Autodesk Inventor part; units mm, degrees
ref_plane "YZ Plane" through (0, 0, 0) normal (1, 0, 0) x (0, 1, 0)
ref_plane "XZ Plane" through (0, 0, 0) normal (0, 1, 0) x (-1, 0, 0)
ref_plane "XY Plane" through (0, 0, 0) normal (0, 0, 1) x (1, 0, 0)
sketch "Sketch1" plane through (0, 0, 0) normal (0, 0, 1) x (1, 0, 0)
  circle A0 centre (0, 0) radius 5.7
  dimension "d0" = 11.4
extrude "Extrusion1" add sketch "Sketch1" along normal blind 3
chamfer "Chamfer1" distance 0.8 angle 45 1 edges at (-5.7, 0, 3)
sketch "Sketch2" plane through (0, 0, 0) normal (0, 0, 1) x (1, 0, 0)
  circle A0 centre (0, 0) radius 2.9
  dimension "d6" = 5.8
extrude "Extrusion2" cut sketch "Sketch2" along normal blind 10
properties part number "Insert3mm"
CAD build for the part. Positions are in the model's coordinates, mm. Coordinates: 2 decimals unless noted, no trailing zeros. Loops run counter-clockwise (first coordinate to the right, second up) from the corner with the lowest first, then second, coordinate; pieces in that order, holes last. Notation, with made-up numbers: (86, 57) - (131, 57) arc R13 ccw to (131, 66) - close; hole circle Ø6 at (-15, 86.5). An arc over 180 degrees is marked (long way). Return JSON: item names as keys, results as strings.
1. Probe L1, parallel to Y at x = 0, z = 1.6; L2, parallel to Y at x = -1, z = 1.6; L3, parallel to X at y = 2.5, z = 0.4. List the from-to ranges inside material, lowest first. Write a range as from..to.
Result:
{"L1": "y = -5.7..-2.9, 2.9..5.7", "L2": "y = -5.61..-2.72, 2.72..5.61", "L3": "x = -5.12..-1.47, 1.47..5.12"}
2. Band-saw the part on A-A (y = 0). Give the cut face in (x, z).
Result:
{"outline": "(-5.7, 0) - (-2.9, 0) - (-2.9, 3) - (-4.9, 3) - (-5.7, 2.2) - close; (2.9, 0) - (5.7, 0) - (5.7, 2.2) - (4.9, 3) - (2.9, 3) - close"}
3. Band-saw the part on C-C (z = 1.4). Give the cut face in (x, y), and give its area (3 significant figures).
Result:
{"outline": "circle Ø11.4 at (0, 0); hole circle Ø5.8 at (0, 0)", "area": "75.6 mm2"}
4. Drop a flat-ended pin along its axis: pin 1 (4.5 mm diameter, centred on x = 0, y = 0, fed in from +Z). Give the stop position or say it passes through.
Result:
{"pin 1": "passes through"}
5. Band-saw the part on D-D (z = 2.35). Give the cut face in (x, y).
Result:
{"outline": "circle Ø11.1 at (0, 0); hole circle Ø5.8 at (0, 0)"}
6. Mould opens along Y. For faces 1 (the flat face through (-3, 1, 0)), 2 (the cylindrical face through (-2.9, -0.1, 1.5)), 3 (the cylindrical face through (-4.5, 3.5, 1.1)) say: released by +Y, released by -Y, zero draft, split by the parting line, or undercut.
Result:
{"face 1": "zero draft", "face 2": "undercut", "face 3": "split by the parting line"}
